CAD build for the part. Positions are in the model's coordinates, mm. Face numbers are marked on the shaded views. A direction names the side the tool comes from. Give positions to 0.01 mm unless a question says otherwise; leave off trailing zeros. Order: outer loops, then holes, each group sorted by start corner. A loop starts at its lowest first (then second) coordinate and runs counter-clockwise, first axis right, second up.
Item 1: Band-saw the part on C-C on x = -3.5. Give the cut face in (y, z) (3 decimals).
Item 2: Band-saw the part on B-B on z = 0. Give the cut face in (x, y) (3 decimals), plus the area to 4 significant figures.
Item 3: Band-saw the part on A-A on y = -3.25. Give the cut face in (x, z) (3 decimals).
Item 4: Two-plate mould, pull along X, no slides. Class the marked faces 1, 2 and 3: released by +X, released by -X, zero draft, split by the parting line, or undercut.
Item 5: Which spindle directions (+Z, -Z, +X, -X, +Y, -Y) get a long thin tool onto all of the face, cutting with end or side? Do the marked faces 4 and 5. Say none if no direction does.
Item 6: Wall check: L1, parallel to X at y = -1.25, z = -5.25; L2, parallel to Y at x = 0.5, z = -2; L3, parallel to Y at x = 2.25, z = 2. Give the ranges that are in metal, low to high.
Item 7: Band-saw the part on D-D on z = -4.25. Give the cut face in (x, y), plus the area to 3 significant figures.
Item 8: Flat gauge pins, fed straight in: P1, Ø2, axis at x = 0.5, y = -4.5, coming from the -Z side; P2, Ø5, axis at x = 0, z = -4, coming from the +Y side. Where does each tip first touch, or does it go through?
```python
from build123d import *

# Parameters (mm, degrees)
SKETCH_2_R          = 3.175
CUT_EXTRUDE_1_DEPTH = 14


with BuildPart() as part:
    # 草图1 → 旋转1 (revolve)
    with BuildSketch(Plane.XY):
        Polygon((6.5, -3.25), (-6.5, -3.25), (-6.5, 3.25), (-5.5, 3.25), (-5.5, 1.25), (1, 1.25), (1, 3.25), (6.5, 3.25), align=None)
    revolve(axis=Axis((-6.5, -3.25, 0), (1, 0, 0)))

    # 草图2 → 切除-拉伸1 (cut, through all)
    with BuildSketch(Plane.ZY.offset(6.5)):
        with Locations((0, -3.25)):
            Circle(SKETCH_2_R)
    extrude(amount=-CUT_EXTRUDE_1_DEPTH, mode=Mode.SUBTRACT)


solid = part.part
```
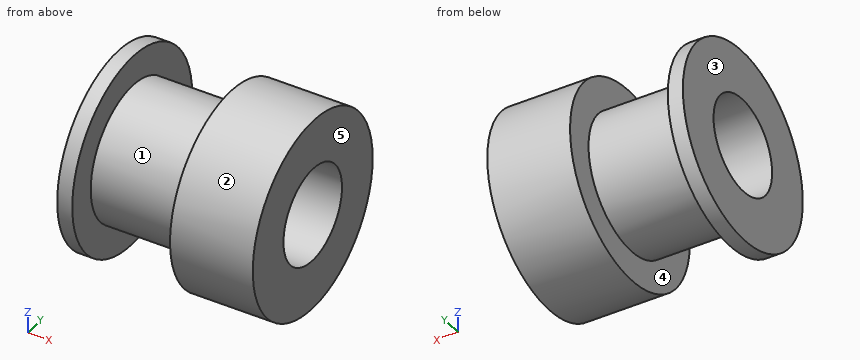
The answers:
1. outline: circle Ø9 at (-3.25, 0); hole circle Ø6.35 at (-3.25, 0)
2. outline: (-6.5, -9.75) - (-5.5, -9.75) - (-5.5, -7.75) - (1, -7.75) - (1, -9.75) - (6.5, -9.75) - (6.5, -6.425) - (-6.5, -6.425) - close; (-6.5, -0.075) - (6.5, -0.075) - (6.5, 3.25) - (1, 3.25) - (1, 1.25) - (-5.5, 1.25) - (-5.5, 3.25) - (-6.5, 3.25) - close
2. area: 60.45 mm2
3. outline: (-6.5, -6.5) - (-5.5, -6.5) - (-5.5, -4.5) - (1, -4.5) - (1, -6.5) - (6.5, -6.5) - (6.5, -3.175) - (-6.5, -3.175) - close; (-6.5, 3.175) - (6.5, 3.175) - (6.5, 6.5) - (1, 6.5) - (1, 4.5) - (-5.5, 4.5) - (-5.5, 6.5) - (-6.5, 6.5) - close
4. face 1: undercut
4. face 2: zero draft
4. face 3: released by -X
5. face 4: none
5. face 5: +Z, -Z, +X, +Y, -Y
6. L1: x = -6.5 to -5.5, 1 to 6.5
6. L2: y = -7.28 to -5.72, -0.78 to 0.78
6. L3: y = -9.43 to -5.72, -0.78 to 2.93
7. outline: (-6.5, -8.17) - (-5.5, -8.17) - (-5.5, -4.73) - (1, -4.73) - (1, -8.17) - (6.5, -8.17) - (6.5, 1.67) - (1, 1.67) - (1, -1.77) - (-5.5, -1.77) - (-5.5, 1.67) - (-6.5, 1.67) - close
7. area: 83.2 mm2
8. P1: stops at z = -6.49
8. P2: stops at y = 3.02
